from build123d import *

# Parameters (mm, degrees)
EXTRUDE_1_DEPTH = 70
SKETCH_4_R      = 1.5
EXTRUDE_2_DEPTH = 6
M3X0_5_1_D      = 2.5
M3X0_5_1_DEPTH  = 7.5
M3X0_5_1_TIP    = 0.751075774


with BuildPart() as part:
    # 草圖1 → 填料-伸長1 (new body)
    with BuildSketch(Plane.XY):
        Polygon((-1.443375673, 2.5), (-2.886751346, 0), (-1.443375673, -2.5), (1.443375673, -2.5), (2.886751346, 0), (1.443375673, 2.5), align=None)
    extrude(amount=EXTRUDE_1_DEPTH)

    # 草圖4 → 填料-伸長2 (add)
    with BuildSketch(Plane(origin=(0, 0, 0), x_dir=(-1, 0, 0), z_dir=(0, 0, -1))):
        Circle(SKETCH_4_R)
    extrude(amount=EXTRUDE_2_DEPTH)

    # M3x0.5 螺紋孔1
    with Locations(Plane.XY.offset(70)):
        with Locations((0, 0)):
            Hole(M3X0_5_1_D / 2, depth=M3X0_5_1_DEPTH)
            with Locations((0, 0, -(M3X0_5_1_DEPTH + M3X0_5_1_TIP / 2))):  # 118° drill point
                Cone(0, M3X0_5_1_D / 2, M3X0_5_1_TIP, mode=Mode.SUBTRACT)


solid = part.part
Verification items for the finished model (mm, model axes). A direction names the side the tool comes from. Coordinates: 2 decimals unless noted, no trailing zeros. One line per item, written item: value. Start each with the question number.
Item 1: Scan lines: probe 1 along X at (y, z) = (0, 67); probe 2 along Y at (x, z) = (0, 66); probe 3 along Z at (x, y) = (1.3, 1.3). Record each from-to range of solid material in increasing order.
Item 2: Mould release check, pull along Y, two halves, no side actions. Record for faces 3 (the flat face through (1, 1, 70)), 4 (the cylindrical face through (0.27, -1.22, 66.2)), 5 (the flat face through (0, -2.5, 35)): released by +Y, released by -Y, zero draft, split by the parting line, or undercut.
Item 3: Access from +Z, -Z, +X, -X, +Y, -Y to the whole of each face (thin tool, end or side, straight path). Record for faces 1 (the flat face through (-2.175, -1.233, 34.51)), 2 (the flat face through (1.24, 1.15, 0)).
Item 4: Gauge pin test, flat end, axial feed: pin 1 (1.5 mm diameter, centred on x = 1.5, y = 1.5, fed in from -Z). Record the tip position at first contact, or that the pin passes through.
Conclusion:
1. probe 1: x = -2.89 to -1.25, 1.25 to 2.89
1. probe 2: y = -2.5 to -1.25, 1.25 to 2.5
1. probe 3: z = 0 to 70
2. face 3: zero draft
2. face 4: undercut
2. face 5: released by -Y
3. face 1: +Z, -Z, -X, -Y
3. face 2: -Z
4. pin 1: stops at z = -6
